Could you check a few things on this model? Use its own coordinates, in mm. A direction names the side the tool comes from. Give positions to 0.01 mm unless a question says otherwise; leave off trailing zeros. Write each loop counter-clockwise with the first axis right and the second up, starting at its lowest first coordinate (ties: lowest second). Pieces come first, ordered by that corner, then holes. Notation, with made-up numbers: (59.25, 31) - (85.25, 31) arc R10 ccw to (85.25, 49) - close; hole circle Ø10 at (57.5, 39). An arc over 180 degrees is marked (long way). Use one line per item in the form item = value.
```python
from build123d import *

# Parameters (mm, degrees)
SKETCH1_W           = 125.73
SKETCH1_H           = 50.8
SKETCH1_W_2         = 113.03
SKETCH1_H_2         = 38.1
BOSS_EXTRUDE1_DEPTH = 76.2
CUT_EXTRUDE1_REACH  = 52.8
SKETCH2_R           = 2.4765
SKETCH2_5_R         = 3.81
CUT_EXTRUDE2_DEPTH  = 51.8
SKETCH5_R           = 3.81
CUT_EXTRUDE4_DEPTH  = 51.8
SKETCH6_R           = 3.81
CUT_EXTRUDE5_DEPTH  = 126.73
SKETCH7_R           = 8.73125
CUT_EXTRUDE6_DEPTH  = 1.984375
SKETCH8_R           = 8.73125
CUT_EXTRUDE7_DEPTH  = 1.984375
SKETCH9_R           = 8.73125
CUT_EXTRUDE8_DEPTH  = 1.984375
SKETCH10_R          = 8.73125
CUT_EXTRUDE9_DEPTH  = 1.984375
SKETCH12_R          = 2.5527
CUT_EXTRUDE11_DEPTH = 7.35


with BuildPart() as part:
    # Sketch1 → Boss-Extrude1 (new body)
    with BuildSketch(Plane(origin=(0, 0, 0), x_dir=(1, 0, 0), z_dir=(0, 1, 0))):
        with Locations((62.865, -25.4)):
            Rectangle(SKETCH1_W, SKETCH1_H)
        with Locations((62.865, -25.4)):
            Rectangle(SKETCH1_W_2, SKETCH1_H_2, mode=Mode.SUBTRACT)
    extrude(amount=BOSS_EXTRUDE1_DEPTH)

    # Sketch2 → Cut-Extrude1 (cut, up to next)
    with BuildSketch(Plane.XY.offset(50.8), mode=Mode.PRIVATE) as cut_extrude1_sk1:
        with Locations((14.526827682, 61.673172318)):
            Circle(SKETCH2_R)
    cut_extrude1_tool1 = extrude(cut_extrude1_sk1.sketch, amount=-CUT_EXTRUDE1_REACH, mode=Mode.PRIVATE) & part.part
    add(cut_extrude1_tool1.solids().sort_by_distance((14.526828, 61.673172, 50.8))[0], mode=Mode.SUBTRACT)
    # Sketch2 → Cut-Extrude1 (cut, up to next)
    with BuildSketch(Plane.XY.offset(50.8), mode=Mode.PRIVATE) as cut_extrude1_sk2:
        with Locations((61.673172318, 61.673172318)):
            Circle(SKETCH2_R)
    cut_extrude1_tool2 = extrude(cut_extrude1_sk2.sketch, amount=-CUT_EXTRUDE1_REACH, mode=Mode.PRIVATE) & part.part
    add(cut_extrude1_tool2.solids().sort_by_distance((61.673172, 61.673172, 50.8))[0], mode=Mode.SUBTRACT)
    # Sketch2 → Cut-Extrude1 (cut, up to next)
    with BuildSketch(Plane.XY.offset(50.8), mode=Mode.PRIVATE) as cut_extrude1_sk3:
        with Locations((61.673172318, 14.526827682)):
            Circle(SKETCH2_R)
    cut_extrude1_tool3 = extrude(cut_extrude1_sk3.sketch, amount=-CUT_EXTRUDE1_REACH, mode=Mode.PRIVATE) & part.part
    add(cut_extrude1_tool3.solids().sort_by_distance((61.673172, 14.526828, 50.8))[0], mode=Mode.SUBTRACT)
    # Sketch2 → Cut-Extrude1 (cut, up to next)
    with BuildSketch(Plane.XY.offset(50.8), mode=Mode.PRIVATE) as cut_extrude1_sk4:
        with Locations((14.526827682, 14.526827682)):
            Circle(SKETCH2_R)
    cut_extrude1_tool4 = extrude(cut_extrude1_sk4.sketch, amount=-CUT_EXTRUDE1_REACH, mode=Mode.PRIVATE) & part.part
    add(cut_extrude1_tool4.solids().sort_by_distance((14.526828, 14.526828, 50.8))[0], mode=Mode.SUBTRACT)

    # Sketch2_5 → Cut-Extrude2 (cut, through all)
    with BuildSketch(Plane.XY.offset(50.8)):
        with Locations((38.1, 38.1)):
            Circle(SKETCH2_5_R)
    extrude(amount=-CUT_EXTRUDE2_DEPTH, mode=Mode.SUBTRACT)

    # Sketch5 → Cut-Extrude4 (cut, through all)
    with BuildSketch(Plane.XY.offset(50.8)):
        with Locations((100.33, 38.1)):
            Circle(SKETCH5_R)
    extrude(amount=-CUT_EXTRUDE4_DEPTH, mode=Mode.SUBTRACT)

    # Sketch6 → Cut-Extrude5 (cut, through all)
    with BuildSketch(Plane.ZY):
        with Locations((25.4, 19.05)):
            Circle(SKETCH6_R)
    extrude(amount=-CUT_EXTRUDE5_DEPTH, mode=Mode.SUBTRACT)

    # Sketch7 → Cut-Extrude6 (cut)
    with BuildSketch(Plane(origin=(6.35, 0, 0), x_dir=(0, 0, -1), z_dir=(1, 0, 0))):
        with Locations((-25.4, 19.05)):
            Circle(SKETCH7_R)
    extrude(amount=-CUT_EXTRUDE6_DEPTH, mode=Mode.SUBTRACT)

    # Sketch8 → Cut-Extrude7 (cut)
    with BuildSketch(Plane(origin=(0, 0, 44.45), x_dir=(-1, 0, 0), z_dir=(0, 0, -1))):
        with Locations((-38.1, 38.1)):
            Circle(SKETCH8_R)
        with Locations((-100.33, 38.1)):
            Circle(SKETCH8_R)
    extrude(amount=-CUT_EXTRUDE7_DEPTH, mode=Mode.SUBTRACT)

    # Sketch9 → Cut-Extrude8 (cut)
    with BuildSketch(Plane.ZY.offset(-119.38)):
        with Locations((25.4, 19.05)):
            Circle(SKETCH9_R)
    extrude(amount=-CUT_EXTRUDE8_DEPTH, mode=Mode.SUBTRACT)

    # Sketch10 → Cut-Extrude9 (cut)
    with BuildSketch(Plane.XY.offset(6.35)):
        with Locations((38.1, 38.1)):
            Circle(SKETCH10_R)
        with Locations((100.33, 38.1)):
            Circle(SKETCH10_R)
    extrude(amount=-CUT_EXTRUDE9_DEPTH, mode=Mode.SUBTRACT)

    # Sketch12 → Cut-Extrude11 (cut, through all)
    with BuildSketch(Plane(origin=(0, 0, 44.45), x_dir=(-1, 0, 0), z_dir=(0, 0, -1))):
        with Locations((-87.63, 9.525)):
            Circle(SKETCH12_R)
        with Locations((-113.03, 9.525)):
            Circle(SKETCH12_R)
        with Locations((-113.03, 66.675)):
            Circle(SKETCH12_R)
        with Locations((-87.63, 66.675)):
            Circle(SKETCH12_R)
    extrude(amount=-CUT_EXTRUDE11_DEPTH, mode=Mode.SUBTRACT)


solid = part.part
```
1. If we mould it in two halves opening along Y, with no side actions, what happens to faces 4 (the face through (46.43, 40.72, 5.37)), 5 (the face through (119.38, 38, 26))? For each: pulls with the +Y half, pulls with the -Y half, needs draft (parallel to the pull), parting line crosses it, or undercut.
Response values:
face_4 = undercut
face_5 = needs draft
2. If I drill on line 1 (Z direction, x = 86.5, y = 64); line 2 (X direction, y = 22.5, z = 27.5), over which ranges is the centre line in solid material (lowest first)? Write a range as from..to.
Response values:
line_1 = 0..6.35, 44.45..50.8
line_2 = 0..4.37, 121.36..125.73
3. Imagine slicing it at B-B, the plane y = 19.05. List the corners of the cut face in (x, z) for me.
Response values:
outline = (0, 0) - (125.73, 0) - (125.73, 21.59) - (121.36, 21.59) - (121.36, 16.67) - (119.38, 16.67) - (119.38, 6.35) - (6.35, 6.35) - (6.35, 16.67) - (4.37, 16.67) - (4.37, 21.59) - (0, 21.59) - close; (0, 29.21) - (4.37, 29.21) - (4.37, 34.13) - (6.35, 34.13) - (6.35, 44.45) - (119.38, 44.45) - (119.38, 34.13) - (121.36, 34.13) - (121.36, 29.21) - (125.73, 29.21) - (125.73, 50.8) - (0, 50.8) - close
4. Imagine slicing it at C-C, the plane x = 75.5. List the corners of the cut face in (y, z) for me, and give its area (3 significant figures).
Response values:
outline = (0, 0) - (76.2, 0) - (76.2, 6.35) - (0, 6.35) - close; (0, 44.45) - (76.2, 44.45) - (76.2, 50.8) - (0, 50.8) - close
area = 968 mm²
5. Which directions (+Z, -Z, +X, -X, +Y, -Y) give clear straight access to the entire face, cutting with the end or side of a thin tool? Please do faces 1 (the face through (42, 36, 4.366)), 2 (the face through (35.08, 35.78, 2.21)), 3 (the face through (115.58, 9.64, 47.58)).
Response values:
face_1 = none
face_2 = +Z, -Z
face_3 = +Z
6. For pin 1 (4 mm diameter, centred on x = 14.53, y = 14.53, fed in from +Z), with a flat end and sliding along its axis, tell me the tip position at first contact or that it passes through.
Response values:
pin_1 = 6.35
7. Imagine slicing it at D-D, the plane y = 52.5. List the corners of the cut face in (x, z) for me, and give its area (3 significant figures).
Response values:
outline = (0, 0) - (125.73, 0) - (125.73, 50.8) - (0, 50.8) - close; hole (6.35, 6.35) - (119.38, 6.35) - (119.38, 44.45) - (6.35, 44.45) - close
area = 2,080 mm²
8. Imagine slicing it at A-A, the plane z = 43. List the corners of the cut face in (x, y) for me, and give its area (3 significant figures).
Response values:
outline = (0, 0) - (6.35, 0) - (6.35, 76.2) - (0, 76.2) - close; (119.38, 0) - (125.73, 0) - (125.73, 76.2) - (119.38, 76.2) - close
area = 968 mm²
